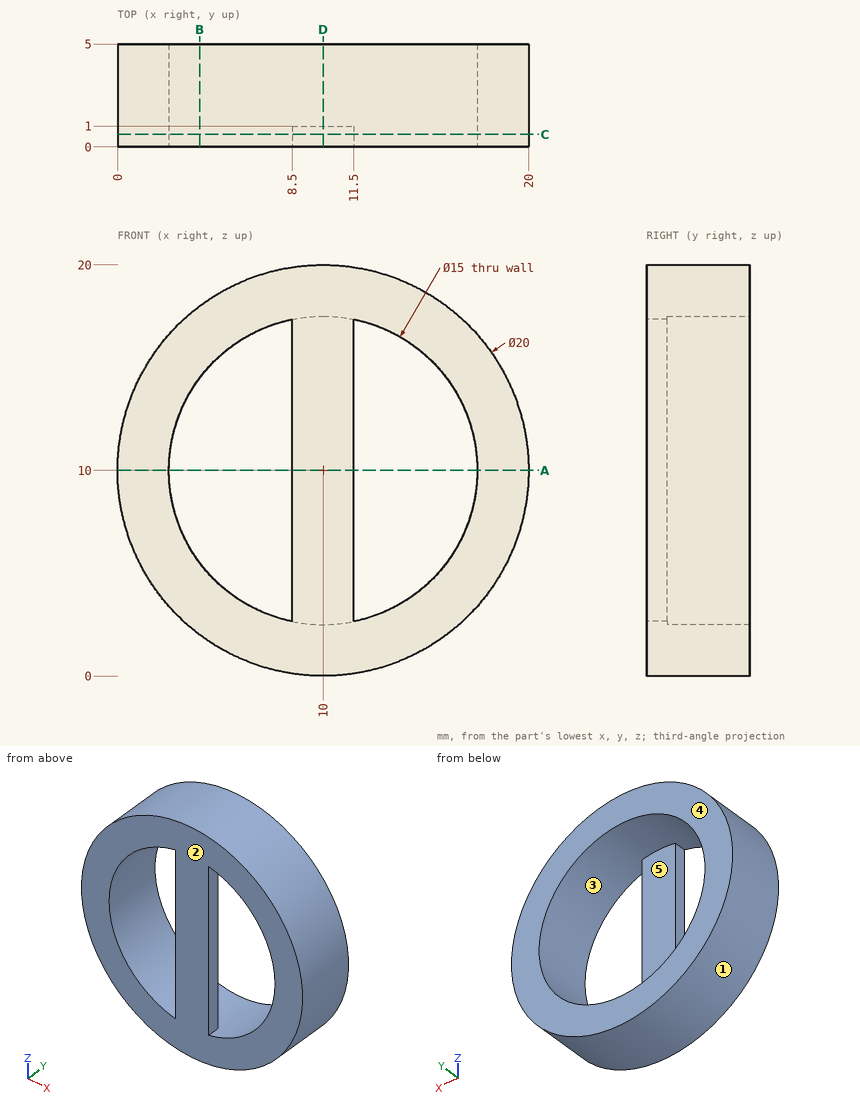
Answer from the drawing. Dimensions are ordinates in mm from the lowest x, y and z of the part. A direction names the side the tool comes from. Give positions to 0.01 mm unless a question says otherwise; leave off trailing zeros. Order: outer loops, then holes, each group sorted by start corner. A loop starts at its lowest first (then second) coordinate and runs counter-clockwise, first axis right, second up.
(1) For the marked faces 4 and 5, determine the directions among +Z, -Z, +X, -X, +Y, -Y from which every point of the face is accessible in a straight line to the end or side of a thin tool.
(2) Find section B-B (x = 4). Give the vertices of the cut face in (y, z).
(3) Given pin 1 (0.8 mm diameter, centred on y = 0.5, z = 8, fed in from -X); pin 2 (1.1 mm diameter, centred on y = 0.5, z = 11, fed in from +X); pin 3 (3 mm diameter, centred on x = 7.5, y = 4, fed in from -Z), each flat-ended and moving along its own axis, determine where each tip first touches the part or whether it passes through.
(4) For a pull along X with two mould halves and no side action, classify the marked faces 1, 2 and 3 as released by +X, released by -X, zero draft, split by the parting line, or undercut.
(5) Find section A-A (z = 10). Give the vertices of the cut face in (x, y).
(6) Find section D-D (x = 10). Give the vertices of the cut face in (y, z), plus the area to 3 significant figures.
(7) Find section C-C (y = 0.6). Give the vertices of the cut face in (x, z), plus the area to 3 significant figures.
(8) Straight lines are drawn through the part: L1, parallel to X at y = 3.25, z = 10; L2, parallel to X at y = 0.95, z = 3.5; L3, parallel to X at y = 0.8, z = 5.5. For each, find the intervals that lie inside material, in ascending order.
Result sheet:
1. face 4: +Z, -Z, +X, -X, +Y
1. face 5: +Y
2. outline: (0, 2) - (5, 2) - (5, 5.5) - (0, 5.5) - close; (0, 14.5) - (5, 14.5) - (5, 18) - (0, 18) - close
3. pin 1: stops at x = 0.13
3. pin 2: stops at x = 19.99
3. pin 3: stops at z = 0.05
4. face 1: split by the parting line
4. face 2: zero draft
4. face 3: undercut
5. outline: (0, 0) - (2.5, 0) - (2.5, 5) - (0, 5) - close; (8.5, 0) - (11.5, 0) - (11.5, 1) - (8.5, 1) - close; (17.5, 0) - (20, 0) - (20, 5) - (17.5, 5) - close
6. outline: (0, 0) - (5, 0) - (5, 2.5) - (1, 2.5) - (1, 17.5) - (5, 17.5) - (5, 20) - (0, 20) - close
6. area: 40.0 mm2
7. outline: circle Ø20 at (10, 10); hole (8.5, 2.65) - (8.5, 17.35) arc R7.5 ccw to start; hole (11.5, 2.65) arc R7.5 ccw to (11.5, 17.35) - close
7. area: 182 mm2
8. L1: x = 0 to 2.5, 17.5 to 20
8. L2: x = 2.4 to 6.26, 8.5 to 11.5, 13.74 to 17.6
8. L3: x = 1.07 to 4, 8.5 to 11.5, 16 to 18.93
